The listing builds one solid part. Answer for the finished solid, in the listing's coordinates (mm). A direction names the side the tool comes from. Round coordinates to 2 decimals unless told otherwise and drop trailing zeros. Write each loop counter-clockwise with the first axis right and the second up, starting at its lowest first coordinate (ties: lowest second). Pieces come first, ordered by that corner, then holes. Notation, with made-up numbers: M 3.5,11.5 L 8.5,11.5 A19 ccw 8.5,22.5 Z; hole C 63,66 d1. An arc over 180 degrees is marked long. Write each question's results on one line, items separated by ' | '.
from build123d import *

# Parameters (mm, degrees)
SKETCH1_W           = 9
SKETCH1_H           = 34.4
SKETCH1_R           = 1.42
BOSS_EXTRUDE1_DEPTH = 40
SKETCH1_3_R         = 1.42
CUT_EXTRUDE1_DEPTH  = 10
SKETCH2_W           = 40
SKETCH2_H           = 3
CUT_EXTRUDE2_DEPTH  = 6
CUT_EXTRUDE3_DEPTH  = 9
CUT_EXTRUDE6_DEPTH  = 7
SKETCH6_R           = 2.0193
CUT_EXTRUDE5_DEPTH  = 20
FILLET2_R           = 0.5
CHAMFER4_SIZE       = 3
FILLET3_R           = 0.5


with BuildPart() as part:
    # Sketch1 → Boss-Extrude1 (new body)
    with BuildSketch(Plane.XY):
        with Locations((4.5, 17.2)):
            Rectangle(SKETCH1_W, SKETCH1_H)
        with Locations((4.5, 15.4)):
            Circle(SKETCH1_R, mode=Mode.SUBTRACT)
        with Locations((4.5, 24.4)):
            Circle(SKETCH1_R, mode=Mode.SUBTRACT)
        with Locations((4.5, 24.4)):
            Circle(SKETCH1_R)
        with Locations((4.5, 15.4)):
            Circle(SKETCH1_R)
        with Locations((4.5, 31.4)):
            Circle(SKETCH1_R)
    extrude(amount=BOSS_EXTRUDE1_DEPTH)

    # Sketch1<3> → Cut-Extrude1 (cut)
    with BuildSketch(Plane.XY):
        with Locations((4.5, 24.4)):
            Circle(SKETCH1_3_R)
        with Locations((4.5, 31.4)):
            Circle(SKETCH1_3_R)
        with Locations((4.5, 15.4)):
            Circle(SKETCH1_3_R)
    extrude(amount=CUT_EXTRUDE1_DEPTH, mode=Mode.SUBTRACT)

    # Sketch2 → Cut-Extrude2 (cut)
    with BuildSketch(Plane(origin=(9, 0, 0), x_dir=(0, 0, -1), z_dir=(1, 0, 0))):
        with Locations((-20, 6.2)):
            Rectangle(SKETCH2_W, SKETCH2_H)
    extrude(amount=-CUT_EXTRUDE2_DEPTH, mode=Mode.SUBTRACT)

    # Sketch3 → Cut-Extrude3 (cut)
    with BuildSketch(Plane(origin=(9, 0, 0), x_dir=(0, 0, -1), z_dir=(1, 0, 0))):
        Polygon((-20, 34.4), (-40, 15), (-48.379363257, 51.913157268), align=None)
    extrude(amount=-CUT_EXTRUDE3_DEPTH, mode=Mode.SUBTRACT)

    # Sketch5 → Cut-Extrude6 (cut)
    with BuildSketch(Plane.ZY.offset(-9)):
        Polygon((20, 34.4), (10, 34.4), (10, 12), (40, 12), (40, 15), align=None)
    extrude(amount=CUT_EXTRUDE6_DEPTH, mode=Mode.SUBTRACT)

    # Sketch6 → Cut-Extrude5 (cut)
    with BuildSketch(Plane.XZ):
        with Locations((6, 35)):
            Circle(SKETCH6_R)
        with Locations((6, 20)):
            Circle(SKETCH6_R)
    extrude(amount=-CUT_EXTRUDE5_DEPTH, mode=Mode.SUBTRACT)

    # Fillet2
    fillet2_edges = [part.edges().sort_by_distance(p)[0] for p in [
        (0, 0, 20),
        (0, 7.5, 40),
        (0, 34.4, 10),
        (0, 24.7, 30),
        (0, 17.2, 0),
    ]]
    fillet(fillet2_edges, radius=FILLET2_R)

    # Chamfer4
    chamfer4_edges = [part.edges().sort_by_distance(p)[0] for p in [
        (9, 2.35, 40),
        (9, 9.85, 40),
    ]]
    chamfer(chamfer4_edges, length=CHAMFER4_SIZE)

    # Fillet3
    fillet3_edges = [part.edges().sort_by_distance(p)[0] for p in [
        (9, 4.7, 18.5),
        (9, 0, 18.5),
        (9, 2.35, 37),
        (9, 9.85, 37),
        (9, 21.05, 0),
        (9, 7.7, 18.5),
        (9, 34.4, 5),
        (9, 12, 23.5),
        (2, 13.5, 40),
        (4, 12, 40),
        (2, 24.7, 30),
        (2, 34.4, 15),
        (9, 23.2, 10),
        (5.5, 34.4, 10),
        (2, 12, 25),
        (2, 23.2, 10),
        (9, 2.35, 0),
    ]]
    fillet(fillet3_edges, radius=FILLET3_R)


solid = part.part
1) The mould has two halves that part along Y. Classify faces 1 (the face through (4.192, 23.014, 4.93)), 2 (the face through (6.932, 2.317, 18.209)), 3 (the face through (0.143, 24.456, 30.035)), 4 (the face through (4.192, 30.014, 4.93)): +Y half, -Y half, draft (parallel to the pull), parting line (faces both ways), or undercut.
Return value:
face 1: undercut | face 2: draft | face 3: +Y half | face 4: undercut
2) Section D-D (x = 7.5) is taken. Determine the outline of the cut face in (y, z), then the cut area to 3 significant figures.
Return value:
outline: M 0,0 L 4.7,0 L 4.7,18.65 L 0,18.65 Z; M 0,21.35 L 4.7,21.35 L 4.7,33.65 L 0,33.65 Z; M 0,36.35 L 4.7,36.35 L 4.7,38.5 L 0,38.5 Z; M 7.7,0 L 34.4,0 L 34.4,9.5 A0.5 ccw 33.9,10 L 12,10 L 12,18.65 L 7.7,18.65 Z; M 7.7,21.35 L 12,21.35 L 12,33.65 L 7.7,33.65 Z; M 7.7,36.35 L 12,36.35 L 12,38.5 L 7.7,38.5 Z | area: 522 mm²
3) Each of these flat-tipped pins is pushed along its axis until it touches: pin 1 (2.5 mm diameter, centred on x = 4.5, y = 24.4, fed in from +Z); pin 2 (1.8 mm diameter, centred on x = 5.5, y = 26, fed in from +Z); pin 3 (4.5 mm diameter, centred on x = 4.5, y = 31.4, fed in from -Z); pin 4 (1.8 mm diameter, centred on x = 5, z = 30, fed in from +Y). Where does it stop, or does it pass through?
Return value:
pin 1: through | pin 2: z = 10 | pin 3: z = 0 | pin 4: y = 12
4) Section C-C (z = 13) is taken. Determine the outline of the cut face in (x, y).
Return value:
outline: M 0,0.5 A0.5 ccw 0.5,0 L 8.5,0 A0.5 ccw 9,0.5 L 9,4.2 A0.5 ccw 8.5,4.7 L 3,4.7 L 3,7.7 L 8.5,7.7 A0.5 ccw 9,8.2 L 9,11.5 A0.5 ccw 8.5,12 L 2.5,12 A0.5 cw 2,12.5 L 2,33.9 A0.5 ccw 1.5,34.4 L 0.5,34.4 A0.5 ccw 0,33.9 Z
5) A tool of negligible diameter and unlimited length cuts with its end or side. For faces 5 (the face through (6.932, 9.82, 18.209)), 6 (the face through (6, 12, 25)), 7 (the face through (3, 6, 20)), from which of +Z, -Z, +X, -X, +Y, -Y can it reach the whole face along a straight path? Write none if from no direction.
Return value:
face 5: +Y, -Y | face 6: +Z, +X, +Y | face 7: +Z, -Z, +X
6) Find the intervals of material crossed by line 1 (Y direction, x = 4.5, z = 7); line 2 (Z direction, x = 6, y = 9.15); line 3 (Y direction, x = 3.75, z = 36), in increasing order.
Return value:
line 1: 0 to 4.7, 7.7 to 13.98, 16.82 to 22.98, 25.82 to 29.98, 32.82 to 34.4 | line 2: 0 to 17.98, 22.02 to 32.98, 37.02 to 40 | line 3: 0 to 4.7, 7.7 to 12
7) Section A-A (z = 4.5) is taken. Determine the outline of the cut face in (x, y), then the cut area to 3 significant figures.
Return value:
outline: M 0,0.5 A0.5 ccw 0.5,0 L 8.5,0 A0.5 ccw 9,0.5 L 9,4.2 A0.5 ccw 8.5,4.7 L 3,4.7 L 3,7.7 L 8.5,7.7 A0.5 ccw 9,8.2 L 9,33.9 A0.5 ccw 8.5,34.4 L 0.5,34.4 A0.5 ccw 0,33.9 Z; hole C 4.5,15.4 d2.84; hole C 4.5,24.4 d2.84; hole C 4.5,31.4 d2.84 | area: 272 mm²
8) Section B-B (y = 13) is taken. Determine the outline of the cut face in (x, z).
Return value:
outline: M 0,0.5 A0.5 ccw 0.5,0 L 8.5,0 A0.5 ccw 9,0.5 L 9,9.5 A0.5 ccw 8.5,10 L 2.5,10 A0.5 cw 2,10.5 L 2,39.5 A0.5 ccw 1.5,40 L 0.5,40 A0.5 ccw 0,39.5 Z
